Job drawing, mm, ordinate dimensions from the low corner. One solid piece. Coordinates: 2 decimals unless noted, no trailing zeros. Write each loop counter-clockwise with the first axis right and the second up, starting at its lowest first coordinate (ties: lowest second). Pieces come first, ordered by that corner, then holes. Notation, with made-up numbers: (80.25, 56) -> (99.25, 56) arc R35 ccw to (99.25, 93) -> close; hole circle Ø1 at (40, -20.75). An arc over 180 degrees is marked (long way). One line per question, with ' | ' between items. Start each with the question number.
Item 1: Saw through at C-C (z = 100). List the corners of the cut face in (x, y).
Item 2: Probe probe 1 along Z at (x, y) = (100, 1.6); probe 2 along X at (y, z) = (1.55, 79); probe 3 along Z at (x, y) = (102, 3.85). List the from-to ranges inside material, lowest first. Write a range as [from, to].
Item 3: Saw through at A-A (x = 80). List the corners of the cut face in (y, z).
Item 4: Saw through at B-B (y = 1.95). Count the separate pieces of the cut face and the enclosed holes in it, and give its area (3 significant figures).
Item 5: Pin check, flat tip, straight feed: pin 1 (4.5 mm diameter, centred on x = 20, z = 40, fed in from +Y). Stop position of the tip, or through.
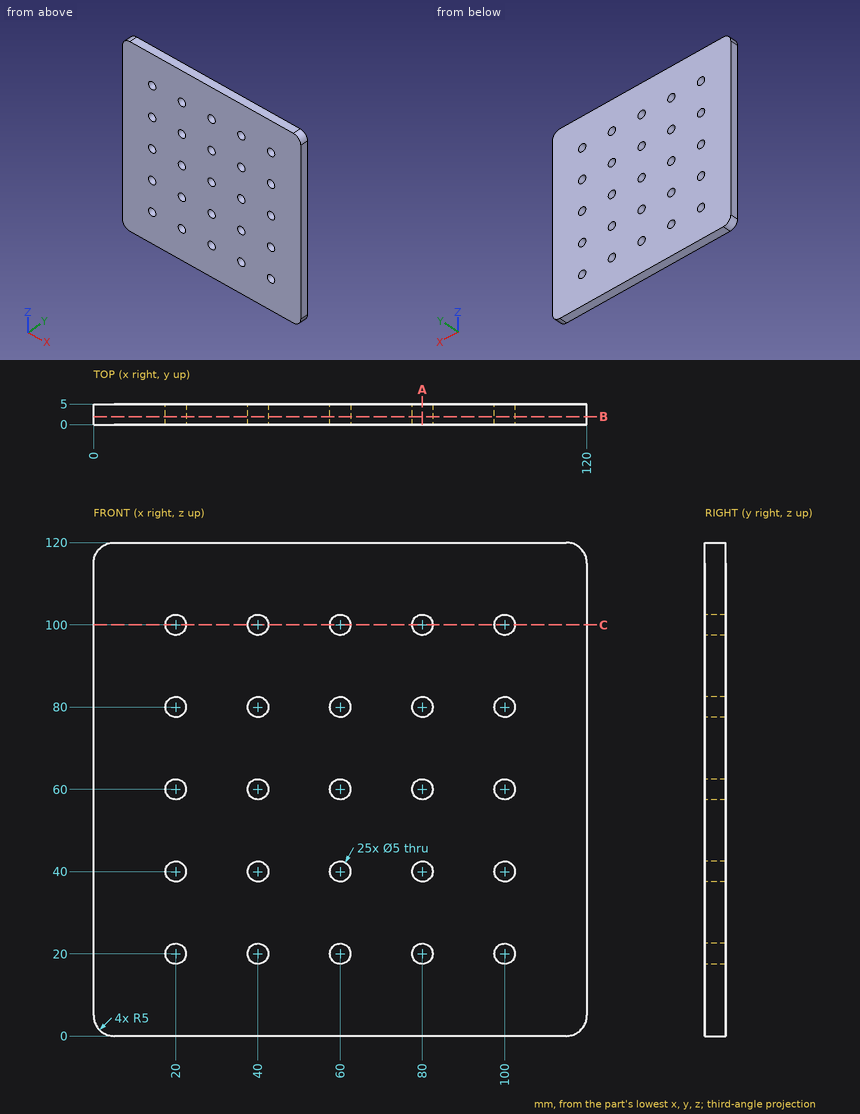
From the geometry:
1) outline: (0, 0) -> (17.5, 0) -> (17.5, 5) -> (0, 5) -> close; (22.5, 0) -> (37.5, 0) -> (37.5, 5) -> (22.5, 5) -> close; (42.5, 0) -> (57.5, 0) -> (57.5, 5) -> (42.5, 5) -> close; (62.5, 0) -> (77.5, 0) -> (77.5, 5) -> (62.5, 5) -> close; (82.5, 0) -> (97.5, 0) -> (97.5, 5) -> (82.5, 5) -> close; (102.5, 0) -> (120, 0) -> (120, 5) -> (102.5, 5) -> close
2) probe 1: [0, 17.5], [22.5, 37.5], [42.5, 57.5], [62.5, 77.5], [82.5, 97.5], [102.5, 120] | probe 2: [0, 17.71], [22.29, 37.71], [42.29, 57.71], [62.29, 77.71], [82.29, 97.71], [102.29, 120] | probe 3: [0, 18.5], [21.5, 38.5], [41.5, 58.5], [61.5, 78.5], [81.5, 98.5], [101.5, 120]
3) outline: (0, 0) -> (5, 0) -> (5, 17.5) -> (0, 17.5) -> close; (0, 22.5) -> (5, 22.5) -> (5, 37.5) -> (0, 37.5) -> close; (0, 42.5) -> (5, 42.5) -> (5, 57.5) -> (0, 57.5) -> close; (0, 62.5) -> (5, 62.5) -> (5, 77.5) -> (0, 77.5) -> close; (0, 82.5) -> (5, 82.5) -> (5, 97.5) -> (0, 97.5) -> close; (0, 102.5) -> (5, 102.5) -> (5, 120) -> (0, 120) -> close
4) separate pieces: 1 | enclosed holes: 25 | area: 13,900 mm2
5) pin 1: through
